```python
from build123d import *

# Parameters (mm, degrees)
F1_DEPTH = 52
F2_R     = 10
F3_DEPTH = 21
F5_DEPTH = 21
F6_R     = 25.99999


# Not quite as in the source:
# - a fillet or chamfer is up to 0.001 mm smaller than in the source, because OpenCascade refuses the exact size


with BuildPart() as f1:
    # F0 (on Front) → F1 (new body)
    with BuildSketch(Plane.XZ):
        Polygon((-69.8465537288, 71.5643691526), (0, 0), (120, 0), (120, 20), (10, 20), (-55.5336798983, 85.5336798983), align=None)
    extrude(amount=-F1_DEPTH)

    # F2 (on face) → F3 (cut)
    with BuildSketch(Plane(origin=(15, 0, 15), x_dir=(0.7071067812, 0, -0.7071067812), z_dir=(0.7071067812, 0, 0.7071067812))):
        with Locations((-73.7496867163, 26)):
            Circle(F2_R)
    extrude(amount=-F3_DEPTH, mode=Mode.SUBTRACT)

    # F4 (on face) → F5 (cut)
    with BuildSketch(Plane.XY.offset(20)):
        with BuildLine():
            ThreePointArc((20, 26), (22.9289321881, 18.9289321881), (30, 16))
            Line((30, 16), (100, 16))
            ThreePointArc((100, 16), (107.0710678119, 18.9289321881), (110, 26))
            ThreePointArc((110, 26), (107.0710678119, 33.0710678119), (100, 36))
            Line((100, 36), (30, 36))
            ThreePointArc((30, 36), (22.9289321881, 33.0710678119), (20, 26))
        make_face()
    extrude(amount=-F5_DEPTH, mode=Mode.SUBTRACT)

    # F6 (radius 26 in the source; OpenCascade refuses exactly that, so slightly less here)
    f6_edges = [f1.edges().sort_by_distance(p)[0] for p in [
        (-62.690117, 0, 78.549025),
        (-62.690117, 52, 78.549025),
    ]]
    fillet(f6_edges, radius=F6_R)


solid = f1.part
```
Geometry check sheet. Reference: the model listing, model coordinates, mm. A direction names the side the tool comes from. Round coordinates to 2 decimals unless told otherwise and drop trailing zeros. Loops run counter-clockwise (first coordinate to the right, second up) from the corner with the lowest first, then second, coordinate; pieces in that order, holes last. Notation, with made-up numbers: (61.25, -33.75) -> (116.25, -33.75) arc R9 cw to (116.25, -20.75) -> close; hole circle Ø5 at (86.25, -40). An arc over 180 degrees is marked (long way). Use a Markdown table: item, result.
(1) Sectioned sample at D-D (z = 22). Enter the section's corners in (x, y).
Calculated:
| item | result |
|---|---|
| outline | (-21.47, 0) -> (8, 0) -> (8, 52) -> (-21.47, 52) -> close |
(2) Sectioned sample at C-C (y = 21.5). Enter the section's corners in (x, z).
Calculated:
| item | result |
|---|---|
| outline | (-69.57, 71.28) -> (-57.75, 59.17) -> (-43.46, 73.46) -> (-55.26, 85.26) -> close; (-45.28, 46.39) -> (0, 0) -> (21.07, 0) -> (21.07, 20) -> (10, 20) -> (-30.83, 60.83) -> close; (108.93, 0) -> (120, 0) -> (120, 20) -> (108.93, 20) -> close |
(3) Set-up check for faces 4 (the flat face through (65, 36, 10)), 5 (the flat face through (-35.41, 25.64, 36.28)), 6 (the flat face through (66, 14, 20)): record each of +Z, -Z, +X, -X, +Y, -Y from which the full face is reachable in a straight line by a thin tool's end or side.
Calculated:
| item | result |
|---|---|
| face 4 | +Z, -Z |
| face 5 | -Z, -X, +Y, -Y |
| face 6 | +Z, +X, +Y, -Y |
(4) Mould release check, pull along X, two halves, no side actions. Record for faces 1 (the flat face through (27, 0, 19)), 2 (the flat face through (65, 16, 10)), 3 (the flat face through (-22, 26, 52)): released by +X, released by -X, zero draft, split by the parting line, or undercut.
Calculated:
| item | result |
|---|---|
| face 1 | zero draft |
| face 2 | undercut |
| face 3 | released by +X |
(5) Go/stop test with flat-tipped pins: P1, Ø6, axis at y = 39.5, z = 65, coming from the +X side; P2, Ø12, axis at x = 79.5, y = 6, coming from the +Z side; P3, Ø10, axis at y = 22.5, z = 28.5, coming from the +X side. Record where each tip stops, or that it passes through.
Calculated:
| item | result |
|---|---|
| P1 | x = -32 |
| P2 | z = 20 |
| P3 | x = 6.5 |
(6) Sectioned sample at A-A (x = 67.5). Enter the section's corners in (y, z), then the cut area to 3 significant figures.
Calculated:
| item | result |
|---|---|
| outline | (0, 0) -> (16, 0) -> (16, 20) -> (0, 20) -> close; (36, 0) -> (52, 0) -> (52, 20) -> (36, 20) -> close |
| area | 640 mm² |
(7) Sectioned sample at B-B (y = 31.5). Enter the section's corners in (x, z).
Calculated:
| item | result |
|---|---|
| outline | (-69.44, 71.14) -> (-57.35, 58.76) -> (-43.05, 73.05) -> (-55.12, 85.12) -> close; (-45.68, 46.81) -> (0, 0) -> (21.65, 0) -> (21.65, 20) -> (10, 20) -> (-31.24, 61.24) -> close; (108.35, 0) -> (120, 0) -> (120, 20) -> (108.35, 20) -> close |
(8) Scan lines: probe 1 along Y at (x, z) = (93, 16); probe 2 along Z at (x, y) = (27.5, 47.5); probe 3 along X at (y, z) = (24, 5). Record each from-to range of solid material in increasing order.
Calculated:
| item | result |
|---|---|
| probe 1 | 0 to 16, 36 to 52 |
| probe 2 | 0 to 20 |
| probe 3 | -4.88 to 20.2, 109.8 to 120 |
